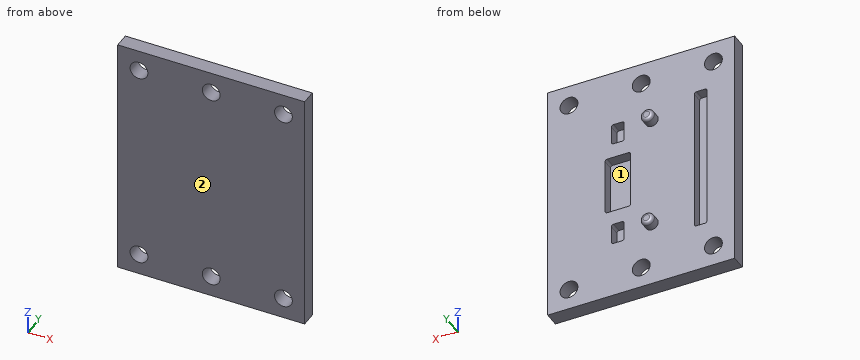
Autodesk Inventor part; units mm, degrees
ref_plane "YZ Plane" through (0, 0, 0) normal (1, 0, 0) x (0, 1, 0)
ref_plane "XZ Plane" through (0, 0, 0) normal (0, 1, 0) x (-1, 0, 0)
ref_plane "XY Plane" through (0, 0, 0) normal (0, 0, 1) x (1, 0, 0)
sketch "Sketch1" plane through (0, 0, 0) normal (0, 1, 0) x (-1, 0, 0)
  line L0 (22, 29) -> (-22, 29)
  line L1 (-22, 29) -> (-22, -29)
  line L2 (-22, -29) -> (22, -29)
  line L3 (22, -29) -> (22, 29)
  point P0 (0, 0)
  point P1 (0, -29)
  dimension "d2" = 44
  dimension "d3" = 58
extrude "Extrusion1" add sketch "Sketch1" along normal blind 3.5
sketch "Sketch2" plane through (0, 3.5, 0) normal (0, 1, 0) x (1, 0, 0)
  line L0 (0, 40.6) -> (0, -40.6)
  line L1 (22, 29) -> (-22, 29)
  point P0 (0, 0)
  point P1 (0, 24)
  dimension "d22" = 5
hole "Hole1" at (0, 3.5, -24) direction (0, -1, 0) diameter 4.2 end through all
pattern_linear "Rectangular Pattern1" count 2 spacing 17 along (-1, 0, 0) count 2 spacing 17 along (1, 0, 0) of "Hole1"
mirror "Mirror1" about plane through (0, 0, 0) normal (0, 0, 1) of "Hole1", "Rectangular Pattern1"
sketch "Sketch3" plane through (0, 3.5, 0) normal (0, 1, 0) x (1, 0, 0)
  circle A0 centre (-2.5, 13.5) radius 1.5
  line L0 (0, 40.6) -> (0, -40.6)
  line L1 (-30.8, 0) -> (30.8, 0)
  circle A1 centre (-2.5, -13.5) radius 1.5
  point P0 (0, 0)
  dimension "d29" = 3
  dimension "d30" = 2.5
  dimension "d31" = 13.5
extrude "Extrusion2" add sketch "Sketch3" along normal blind 2.5
fillet "Fillet1" radius 0.75 2 edges at (-4, 6, -13.5) (-4, 6, 13.5)
sketch "Sketch4" plane through (0, 0, 0) normal (0, 0, 1) x (1, 0, 0)
  line L0 (-15.5, 3.5) -> (-12.5, 3.5)
  line L1 (-12.5, 3.5) -> (-12.5, 1)
  line L2 (-12.5, 1) -> (-15.5, 1)
  line L3 (-15.5, 1) -> (-15.5, 3.5)
  line L4 (-22, 3.5) -> (22, 3.5)
  point P0 (0, 0)
  point P1 (0, 3.5)
  point P2 (-14, 3.5)
  dimension "d35" = 2.5
  dimension "d36" = 3
  dimension "d39" = 14
extrude "Extrusion3" cut sketch "Sketch4" along normal mid plane 35
sketch "Sketch5" plane through (0, 0, 0) normal (0, 0, 1) x (1, 0, 0)
  line L0 (2.5, 3.5) -> (8.5, 3.5)
  line L1 (8.5, 3.5) -> (8.5, 1)
  line L2 (8.5, 1) -> (2.5, 1)
  line L3 (2.5, 1) -> (2.5, 3.5)
  line L4 (-22, 3.5) -> (22, 3.5)
  line L5 (-2.5, 7.2) -> (-2.5, -1.2)
  point P0 (0, 0)
  point P1 (5.5, 3.5)
  dimension "d40" = 6
  dimension "d41" = 2.5
  dimension "d42" = 8
extrude "Extrusion4" cut sketch "Sketch5" along normal mid plane 14
sketch "Sketch6" plane through (0, 3.5, 0) normal (0, 1, 0) x (1, 0, 0)
  line L0 (7, -10.5) -> (4, -10.5)
  line L1 (4, -10.5) -> (4, -15.5)
  line L2 (4, -15.5) -> (7, -15.5)
  line L3 (7, -15.5) -> (7, -10.5)
  line L4 (8.5, 7) -> (8.5, -7)
  line L5 (8.5, -7) -> (2.5, -7)
  point P0 (0, 0)
  point P1 (5.5, -10.5)
  dimension "d45" = 3
  dimension "d46" = 5
  dimension "d47" = 3
  dimension "d48" = 3.5
extrude "Extrusion5" cut sketch "Sketch6" against normal blind 2.5
mirror "Mirror2" about plane through (0, 0, 0) normal (0, 0, 1) of "Extrusion5"
fillet "Fillet2" radius 0.5 16 edges at (-15.5, 2.25, -17.5) (-12.5, 2.25, -17.5) (-15.5, 2.25, 17.5) (-12.5, 2.25, 17.5) (2.5, 2.25, 7) (8.5, 2.25, 7) (7, 2.25, 15.5) (7, 2.25, -10.5) (7, 2.25, 10.5) (8.5, 2.25, -7) (7, 2.25, -15.5) (2.5, 2.25, -7) (4, 2.25, -15.5) (4, 2.25, -10.5) (4, 2.25, 15.5) (4, 2.25, 10.5)
properties part number "connector-houseing-bottom-plate"
Build history of the part. All positions in model axes, mm. Face numbers are marked on the shaded views. Coordinates: 2 decimals unless noted, no trailing zeros. Order: outer loops, then holes, each group sorted by start corner. A loop starts at its lowest first (then second) coordinate and runs counter-clockwise, first axis right, second up. Notation, with made-up numbers: (26, -9.5) -> (60, -9.5) arc R31 cw to (60, 22.5) -> close; hole circle Ø5 at (-5, -19). An arc over 180 degrees is marked (long way). One line per item, written item: value.
(1) Slice it at D-D, the plane y = 1.75. Count the separate pieces of the cut face and the enclosed holes in it, plus the area to 3 significant figures.
Checked values:
separate pieces: 1
enclosed holes: 10
area: 2,250 mm2
(2) Slice it at C-C, the plane z = 4. List the corners of the cut face in (x, y).
Checked values:
outline: (-22, 0) -> (22, 0) -> (22, 3.5) -> (8.5, 3.5) -> (8.5, 1) -> (2.5, 1) -> (2.5, 3.5) -> (-12.5, 3.5) -> (-12.5, 1) -> (-15.5, 1) -> (-15.5, 3.5) -> (-22, 3.5) -> close
(3) Drop flat-ended pins along their axis: pin 1 Ø2.5 at (x, z) = (5.5, -13) entering from +Y; pin 2 Ø4 at (x, z) = (-6, -18) entering from +Y. Give the stop position or say it passes through.
Checked values:
pin 1: y = 1
pin 2: y = 3.5
(4) Probe line 1 (Z direction, x = 0, y = 2.45); line 2 (X direction, y = 2.3, z = -24); line 3 (X direction, y = 1.9, z = -1.5). List the from-to ranges inside material, lowest first. Write a range as [from, to].
Checked values:
line 1: [-29, -26.1], [-21.9, 21.9], [26.1, 29]
line 2: [-22, -19.1], [-14.9, -2.1], [2.1, 14.9], [19.1, 22]
line 3: [-22, -15.5], [-12.5, 2.5], [8.5, 22]
(5) Slice it at A-A, the plane z = -24. List the corners of the cut face in (x, y), plus the area to 3 significant figures.
Checked values:
outline: (-22, 0) -> (-19.1, 0) -> (-19.1, 3.5) -> (-22, 3.5) -> close; (-14.9, 0) -> (-2.1, 0) -> (-2.1, 3.5) -> (-14.9, 3.5) -> close; (2.1, 0) -> (14.9, 0) -> (14.9, 3.5) -> (2.1, 3.5) -> close; (19.1, 0) -> (22, 0) -> (22, 3.5) -> (19.1, 3.5) -> close
area: 110 mm2
(6) Slice it at B-B, the plane x = 17. List the corners of the cut face in (y, z), plus the area to 3 significant figures.
Checked values:
outline: (0, -29) -> (3.5, -29) -> (3.5, -26.1) -> (0, -26.1) -> close; (0, -21.9) -> (3.5, -21.9) -> (3.5, 21.9) -> (0, 21.9) -> close; (0, 26.1) -> (3.5, 26.1) -> (3.5, 29) -> (0, 29) -> close
area: 174 mm2
(7) Mould opens along Z. For the marked faces 1 and 2 say: pulls with the +Z half, pulls with the -Z half, needs draft (parallel to the pull), parting line crosses it, or undercut.
Checked values:
face 1: undercut
face 2: needs draft
